Source: CAD feature listing. Evaluate the final solid. Frame: model axes, mm. Face numbers are marked on the shaded views. A direction names the side the tool comes from. Coordinates: 2 decimals unless noted, no trailing zeros. Order: outer loops, then holes, each group sorted by start corner. A loop starts at its lowest first (then second) coordinate and runs counter-clockwise, first axis right, second up.
```python
from build123d import *

# Parameters (mm, degrees)
F0_R     = 17.5
F1_DEPTH = 2.00000108
F2_R     = 2.5
F3_DEPTH = 6
F6_DEPTH = 8.00100108
F7_R     = 4.1497915573
F7_R_2   = 2.5
F8_DEPTH = 6


# Not quite as in the source:
# - a feature of the source that left no trace in its solid (it failed there, or was rolled back) is left out
# - a feature names something its author has since deleted; it is built from what else it names
# - the program builds the solid bodies; features that only make, move or delete a surface that nothing else refers to are left out


with BuildPart() as f1:
    # F0 (on Front) → F1 (new body)
    with BuildSketch(Plane.XZ):
        with Locations((-15.6701616943, 19.357258454)):
            Circle(F0_R)
    extrude(amount=F1_DEPTH)

    # F2 (on face) → F3 (join)
    with BuildSketch(Plane.XZ.offset(2.00000108)):
        with Locations((-15.6701616943, 19.357258454)):
            Circle(F2_R)
    extrude(amount=F3_DEPTH)

    # F6 (cut, through all): a face of the model
    f6_faces = [f1.faces().sort_by_distance(p)[0] for p in [
        (-15.6701616943, -8.00000108, 19.357258454),
    ]]
    extrude(f6_faces, amount=-F6_DEPTH, mode=Mode.SUBTRACT)

    # F7 (on face) → F8 (join)
    with BuildSketch(Plane.XZ.offset(2.00000108)):
        with Locations((-15.6701616943, 19.357258454)):
            Circle(F7_R)
        with Locations((-15.6701616943, 19.357258454)):
            Circle(F7_R_2, mode=Mode.SUBTRACT)
    extrude(amount=F8_DEPTH)


solid = f1.part
```
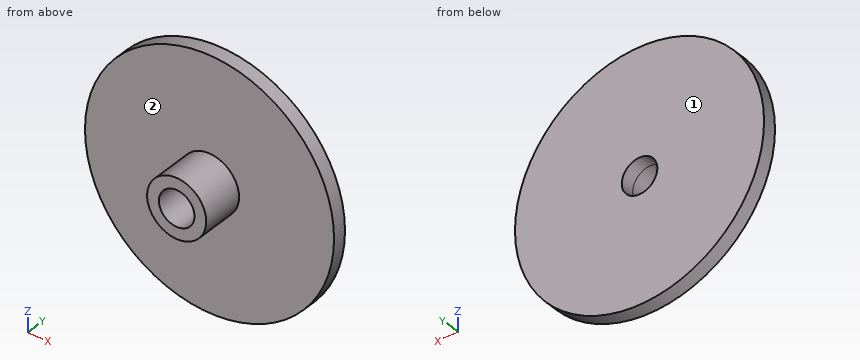
1. Access query for the marked faces 1 and 2. Directions: +Z, -Z, +X, -X, +Y, -Y. A direction counts if a zero-diameter tool reaches every point of the face in a straight line with its end or side. Return the directions, or none.
2. Section query B-B, the plane x = -15. Output: boundary loops of the cut face in (y, z).
3. Material intervals for line 1 along Y through (x, z) = (-16, 28); line 2 along Z through (x, y) = (-16, -1); line 3 along Z through (x, y) = (-16, -2.5), sorted ascending.
4. Section query A-A, the plane z = 21. Output: boundary loops of the cut face in (x, y).
5. Contact query for flat-ended pins moving along their axis: P1, Ø4, axis at x = -18, y = -5, coming from the +Z side; P2, Ø2, axis at y = -6.5, z = 19.5, coming from the -X side; P3, Ø4, axis at y = -4.5, z = 33, coming from the +X side; P4, Ø6, axis at x = -24, z = 8, coming from the -Y side. Output: stop coordinate, or through.
6. Section query C-C, the plane y = -7.25. Output: boundary loops of the cut face in (x, z).
7. Section query D-D, the plane x = -19. Output: boundary loops of the cut face in (y, z).
Answer key:
1. face 1: +Z, -Z, +X, -X, +Y
1. face 2: -Y
2. outline: (-8, 15.26) - (-2, 15.26) - (-2, 1.87) - (0, 1.87) - (0, 16.95) - (-8, 16.95) - close; (-8, 21.77) - (0, 21.77) - (0, 36.84) - (-2, 36.84) - (-2, 23.45) - (-8, 23.45) - close
3. line 1: y = -2 to 0
3. line 2: z = 1.86 to 16.88, 21.84 to 36.85
3. line 3: z = 15.22 to 16.88, 21.84 to 23.49
4. outline: (-33.09, -2) - (-19.48, -2) - (-19.48, -8) - (-17.55, -8) - (-17.55, 0) - (-33.09, 0) - close; (-13.79, -8) - (-11.86, -8) - (-11.86, -2) - (1.75, -2) - (1.75, 0) - (-13.79, 0) - close
5. P1: stops at z = 23.49
5. P2: stops at x = -19.82
5. P3: passes through
5. P4: stops at y = -2
6. outline: circle Ø8.3 at (-15.67, 19.36); hole circle Ø5 at (-15.67, 19.36)
7. outline: (-8, 16.88) - (-2, 16.88) - (-2, 2.18) - (0, 2.18) - (0, 36.54) - (-2, 36.54) - (-2, 21.83) - (-8, 21.83) - close
